Design review of the part built by this model. Coordinates are the model's own, in mm. Face numbers are marked on the shaded views. Coordinates: 2 decimals unless noted, no trailing zeros. Order: outer loops, then holes, each group sorted by start corner. A loop starts at its lowest first (then second) coordinate and runs counter-clockwise, first axis right, second up. Notation, with made-up numbers: M 48.25,31.25 L 63.25,31.25 A17 cw 63.25,41.25 Z; hole C 83.5,-28 d1. An arc over 180 degrees is marked long. Use CSV: the item, a comma, the result in double quotes.
```python
from build123d import *

# Parameters (mm, degrees)
SKETCH1_W           = 32
SKETCH1_H           = 40
EXTRUDE1_DEPTH      = 6
SKETCH8_R           = 6
CUT_EXTRUDE6_DEPTH  = 6
SKETCH5_R           = 1.5
CUT_EXTRUDE4_DEPTH  = 6
CIRPATTERN1_COUNT   = 3
CUT_EXTRUDE13_DEPTH = 3
SKETCH20_R          = 4
CUT_EXTRUDE14_DEPTH = 3
SKETCH25_R          = 1.25
EXTRUDE4_DEPTH      = 3
SKETCH29_R          = 1.25
EXTRUDE7_DEPTH      = 10
EXTRUDE13_START     = -10
SKETCH27_R          = 1.25
EXTRUDE13_DEPTH     = 10


# Read off the part's stored shape, not the designer's step: M3 Tapped Hole2
with BuildPart() as part:
    # Sketch1 → Extrude1 (new body)
    with BuildSketch(Plane.XY):
        Rectangle(SKETCH1_W, SKETCH1_H)
    extrude(amount=-EXTRUDE1_DEPTH)

    # Sketch8 → Cut-Extrude6 (cut)
    with BuildSketch(Plane(origin=(0, 0, -6), x_dir=(-1, 0, 0), z_dir=(0, 0, -1))):
        with Locations((0, 11)):
            Circle(SKETCH8_R)
    extrude(amount=-CUT_EXTRUDE6_DEPTH, mode=Mode.SUBTRACT)

    # Sketch5 → Cut-Extrude4 (cut)
    with BuildSketch(Plane(origin=(0, 0, -6), x_dir=(-1, 0, 0), z_dir=(0, 0, -1))):
        Circle(SKETCH5_R)
    cut_extrude4 = extrude(amount=-CUT_EXTRUDE4_DEPTH, mode=Mode.SUBTRACT)

    # CirPattern1: Cut-Extrude4 ×3 about axis
    cirpattern1_axis = Axis((0, 11, 0), (0, 0, 1))
    for i in range(1, CIRPATTERN1_COUNT):
        add(cut_extrude4.rotate(cirpattern1_axis, i * 360 / CIRPATTERN1_COUNT), mode=Mode.SUBTRACT)

    # Sketch19 → Cut-Extrude13 (cut)
    with BuildSketch(Plane(origin=(0, 0, -6), x_dir=(-1, 0, 0), z_dir=(0, 0, -1))):
        with BuildLine():
            Line((10, 4), (0, 4))
            ThreePointArc((0, 4), (-2.828427125, 2.828427125), (-4, 0))
            Line((-4, 0), (-4, -10))
            Line((-4, -10), (0, -10))
            ThreePointArc((0, -10), (7.071067812, -7.071067812), (10, 0))
            Line((10, 0), (10, 4))
        make_face()
    extrude(amount=-CUT_EXTRUDE13_DEPTH, mode=Mode.SUBTRACT)

    # Sketch20 → Cut-Extrude14 (cut)
    with BuildSketch(Plane(origin=(0, 0, -3), x_dir=(-1, 0, 0), z_dir=(0, 0, -1))):
        with Locations(Location((0, 0, 0), (0, 0, 180))):
            Circle(SKETCH20_R)
    extrude(amount=-CUT_EXTRUDE14_DEPTH, mode=Mode.SUBTRACT)

    # Sketch25 → Extrude4 (cut)
    with BuildSketch(Plane(origin=(0, 0, -3), x_dir=(-1, 0, 0), z_dir=(0, 0, -1))):
        with Locations((-1, -7)):
            Circle(SKETCH25_R)
        with Locations((7, 1)):
            Circle(SKETCH25_R)
    extrude(amount=-EXTRUDE4_DEPTH, mode=Mode.SUBTRACT)

    # Sketch29 → Extrude7 (cut)
    with BuildSketch(Plane.XZ.offset(20)):
        with Locations(Location((-13, -3, 0), (0, 0, 270))):
            Circle(SKETCH29_R)
        with Locations(Location((13, -3, 0), (0, 0, 270))):
            Circle(SKETCH29_R)
    extrude(amount=-EXTRUDE7_DEPTH, mode=Mode.SUBTRACT)

    # Sketch27 → Extrude13 (cut)
    with BuildSketch(Plane(origin=(0, 20, 0), x_dir=(1, 0, 0), z_dir=(0, 1, 0)).offset(EXTRUDE13_START)):
        with Locations(Location((-13, 3, 0), (0, 0, 90))):
            Circle(SKETCH27_R)
        with Locations(Location((13, 3, 0), (0, 0, 90))):
            Circle(SKETCH27_R)
    extrude(amount=EXTRUDE13_DEPTH, mode=Mode.SUBTRACT)

    # M3 Tapped Hole2 outline → M3 Tapped Hole2 (revolve, cut)
    with BuildSketch(Plane(origin=(13, 0, -3), x_dir=(1, 0, 0), z_dir=(0, 0, 1))):
        Polygon((1.25, -10), (0, -9.248924226), (0, -10), align=None)
        Polygon((0, 10), (0, 9.248924226), (1.25, 10), align=None)
    revolve(axis=Axis((13, 0, -3), (0, 1, 0)), mode=Mode.SUBTRACT)

    # M3 Tapped Hole2 2 outline → M3 Tapped Hole2 2 (revolve, cut)
    with BuildSketch(Plane(origin=(-13, 0, -3), x_dir=(1, 0, 0), z_dir=(0, 0, 1))):
        Polygon((1.25, -10), (0, -9.248924226), (0, -10), align=None)
        Polygon((0, 10), (0, 9.248924226), (1.25, 10), align=None)
    revolve(axis=Axis((-13, 0, -3), (0, 1, 0)), mode=Mode.SUBTRACT)


solid = part.part
```
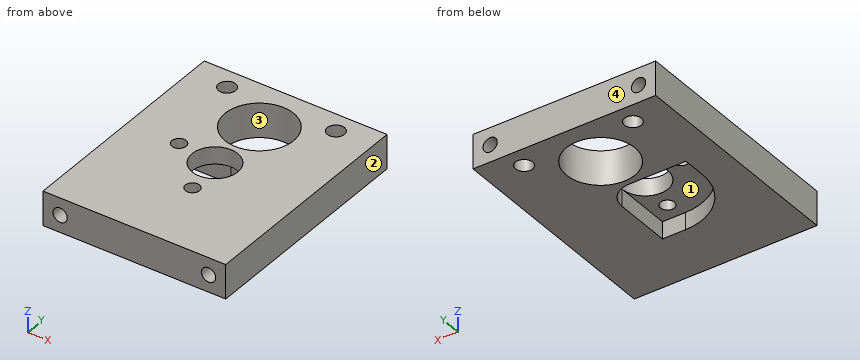
(1) Clearance check with flat-ended pins moving along their axes: P1, Ø2, axis at x = -13, z = -3, coming from the -Y side; P2, Ø1.5, axis at x = 13, z = -3, coming from the -Y side; P3, Ø1.5, axis at x = 13, z = -3, coming from the +Y side. State where each tip first meets the part, or that it passes through.
The answers:
P1,"stops at y = -9.85"
P2,"stops at y = -9.7"
P3,"stops at y = 9.7"
(2) Add section A-A on y = 11. State the section outline as (x, z) points, and give its area (3 significant figures).
The answers:
outline,"M -16,-6 L -6,-6 L -6,0 L -16,0 Z; M 6,-6 L 16,-6 L 16,0 L 6,0 Z; hole C -13,-3 d2.5; hole C 13,-3 d2.5"
area,"110 mm2"
(3) Add section B-B on y = 16.5. State the section outline as (x, z) points, and give its area (3 significant figures).
The answers:
outline,"M -16,-6 L -11.03,-6 L -11.03,0 L -16,0 Z; M -8.03,-6 L -2.4,-6 L -2.4,0 L -8.03,0 Z; M 2.4,-6 L 8.03,-6 L 8.03,0 L 2.4,0 Z; M 11.03,-6 L 16,-6 L 16,0 L 11.03,0 Z; hole C -13,-3 d2.5; hole C 13,-3 d2.5"
area,"117 mm2"
(4) Add section C-C on x = 1. State the section outline as (y, z) points, and give its area (4 significant figures).
The answers:
outline,"M -20,-6 L -10,-6 L -10,-3 L -8.25,-3 L -8.25,0 L -20,0 Z; M -5.75,-3 L -3.87,-3 L -3.87,0 L -5.75,0 Z; M 3.87,-6 L 5.08,-6 L 5.08,0 L 3.87,0 Z; M 16.92,-6 L 20,-6 L 20,0 L 16.92,0 Z"
area,"96.65 mm2"
(5) The part is to be moulded in two halves that separate along Y. For the marked faces 1, 2, 3 and 4, say which applies: pulls with the +Y half, pulls with the -Y half, needs draft (parallel to the pull), parting line crosses it, or undercut.
The answers:
face 1,"undercut"
face 2,"needs draft"
face 3,"undercut"
face 4,"pulls with the +Y half"
(6) Wall thickness on probe 1 along Y at (x, z) = (0, -5.25); probe 2 along X at (y, z) = (-16.5, -3); probe 3 along Y at (x, z) = (0, -1.25): over which ranges is each line inside the solid? List them lowest first.
The answers:
probe 1,"y = -20 to -10, 4 to 5, 17 to 20"
probe 2,"x = -16 to -14.25, -11.75 to 11.75, 14.25 to 16"
probe 3,"y = -20 to -7.75, -6.25 to -4, 4 to 5, 17 to 20"
(7) Add section D-D on y = -7. State the section outline as (x, z) points, and give its area (3 significant figures).
The answers:
outline,"M -16,-6 L -7.14,-6 L -7.14,-3 L -0.25,-3 L -0.25,0 L -16,0 Z; M 2.25,-3 L 4,-3 L 4,-6 L 16,-6 L 16,0 L 2.25,0 Z"
area,"151 mm2"
